from build123d import *

# Parameters (mm, degrees)
SM_BASE_FLANGE_1_DEPTH = 24
CUT_EXTRUDE_1_DEPTH    = 135.033577883
FILLET_1_R             = 10


# Sheet-metal steps are written as plain solids
with BuildPart() as part:
    # Sketch 1 → 基体-法兰1 (new, symmetric)
    with BuildSketch(Plane(origin=(0, 0, 0), x_dir=(0, 0, -1), z_dir=(1, 0, 0))):
        with BuildLine():
            Line((-125, 50), (-125, 16))
            ThreePointArc((-125, 16), (-120.313708499, 4.686291501), (-109, 0))
            Line((-109, 0), (109, 0))
            ThreePointArc((109, 0), (120.313708499, 4.686291501), (125, 16))
            Line((125, 16), (125, 50))
            Line((125, 50), (117, 50))
            Line((117, 50), (117, 16))
            ThreePointArc((117, 16), (114.656854249, 10.343145751), (109, 8))
            Line((109, 8), (-109, 8))
            ThreePointArc((-109, 8), (-114.656854249, 10.343145751), (-117, 16))
            Line((-117, 16), (-117, 50))
            Line((-117, 50), (-125, 50))
        make_face()
    extrude(amount=SM_BASE_FLANGE_1_DEPTH, both=True)

    # 草图6 → 切除-拉伸1 (cut, through all)
    with BuildSketch(Plane(origin=(0, 8, 0), x_dir=(1, 0, 0), z_dir=(0, 1, 0))):
        with BuildLine():
            Line((7.5, 77.5), (7.5, 72.5))
            ThreePointArc((7.5, 72.5), (0, 65), (-7.5, 72.5))
            Line((-7.5, 72.5), (-7.5, 77.5))
            ThreePointArc((-7.5, 77.5), (0, 85), (7.5, 77.5))
        make_face()
        with BuildLine():
            Line((7.5, 27.5), (7.5, 22.5))
            ThreePointArc((7.5, 22.5), (0, 15), (-7.5, 22.5))
            Line((-7.5, 22.5), (-7.5, 27.5))
            ThreePointArc((-7.5, 27.5), (0, 35), (7.5, 27.5))
        make_face()
        with BuildLine():
            Line((7.5, -22.5), (7.5, -27.5))
            ThreePointArc((7.5, -27.5), (0, -35), (-7.5, -27.5))
            Line((-7.5, -27.5), (-7.5, -22.5))
            ThreePointArc((-7.5, -22.5), (0, -15), (7.5, -22.5))
        make_face()
        with BuildLine():
            Line((7.5, -72.5), (7.5, -77.5))
            ThreePointArc((7.5, -77.5), (0, -85), (-7.5, -77.5))
            Line((-7.5, -77.5), (-7.5, -72.5))
            ThreePointArc((-7.5, -72.5), (0, -65), (7.5, -72.5))
        make_face()
    extrude(amount=-CUT_EXTRUDE_1_DEPTH, mode=Mode.SUBTRACT)

    # 圆角1
    fillet_1_edges = [part.edges().sort_by_distance(p)[0] for p in [
        (-24, 50, 121),
        (-24, 50, -121),
        (24, 50, 121),
        (24, 50, -121),
    ]]
    fillet(fillet_1_edges, radius=FILLET_1_R)


solid = part.part
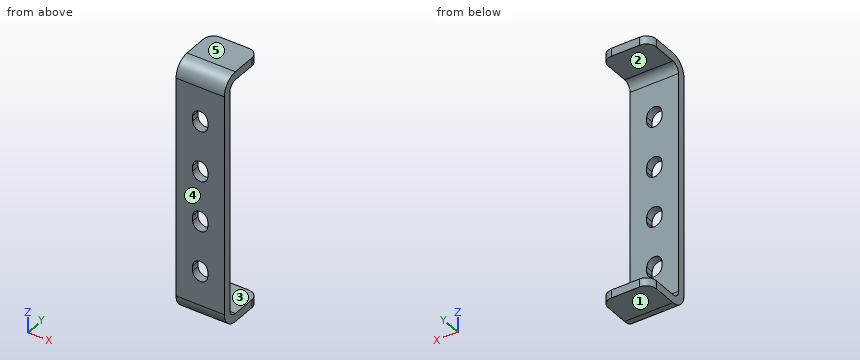
The listing builds one solid part. Answer for the finished solid, in the listing's coordinates (mm). Face numbers are marked on the shaded views. A direction names the side the tool comes from. Round coordinates to 2 decimals unless told otherwise and drop trailing zeros. Order: outer loops, then holes, each group sorted by start corner. A loop starts at its lowest first (then second) coordinate and runs counter-clockwise, first axis right, second up. Notation, with made-up numbers: (41, -4.5) -> (63, -4.5) arc R16 ccw to (63, 4.5) -> close; hole circle Ø1 at (-32.5, 66). An arc over 180 degrees is marked (long way). One line per item, written item: value.
Item 1: Straight lines are drawn through the part: L1, parallel to Z at x = -4, y = 18; L2, parallel to Z at x = 2.5, y = 2; L3, parallel to Y at x = 18, z = 97.5. For each, find the intervals that lie inside material, in ascending order.
Taken from the geometry:
L1: z = -125 to -117, 117 to 125
L2: z = -116.75 to -84.57, -65.43 to -34.57, -15.43 to 15.43, 34.57 to 65.43, 84.57 to 116.75
L3: y = 0 to 8
Item 2: Find section C-C, the plane z = -30. Give the vertices of the cut face in (x, y).
Taken from the geometry:
outline: (-24, 0) -> (-7.07, 0) -> (-7.07, 8) -> (-24, 8) -> close; (7.07, 0) -> (24, 0) -> (24, 8) -> (7.07, 8) -> close
Item 3: For a pull along Z with two mould halves and no side action, classify the marked faces 3, 4 and 5 as released by +Z, released by -Z, zero draft, split by the parting line, or undercut.
Taken from the geometry:
face 3: undercut
face 4: zero draft
face 5: released by +Z
Item 4: Given P1, Ø10, axis at x = -1, z = -24.5, coming from the +Y side; P2, Ø3, axis at x = 6.5, y = 9, coming from the +Z side (3 decimals); P3, Ø8, axis at x = -16, y = 10, coming from the +Z side; P4, Ø6, axis at x = -13.5, z = 21.5, coming from the +Y side, each flat-ended and moving along its own axis, determine where each tip first touches the part or whether it passes through.
Taken from the geometry:
P1: passes through
P2: stops at z = 124.025
P3: stops at z = 124.87
P4: stops at y = 8
Item 5: Find section A-A, the plane x = 0. Give the vertices of the cut face in (y, z).
Taken from the geometry:
outline: (0, -109) arc R16 ccw to (16, -125) -> (50, -125) -> (50, -117) -> (16, -117) arc R8 cw to (8, -109) -> (8, -85) -> (0, -85) -> close; (0, -65) -> (8, -65) -> (8, -35) -> (0, -35) -> close; (0, -15) -> (8, -15) -> (8, 15) -> (0, 15) -> close; (0, 35) -> (8, 35) -> (8, 65) -> (0, 65) -> close; (0, 85) -> (8, 85) -> (8, 109) arc R8 cw to (16, 117) -> (50, 117) -> (50, 125) -> (16, 125) arc R16 ccw to (0, 109) -> close
Item 6: For the marked faces 1 and 2, determine the directions among +Z, -Z, +X, -X, +Y, -Y from which every point of the face is accessible in a straight line to the end or side of a thin tool.
Taken from the geometry:
face 1: -Z, +X, -X, +Y, -Y
face 2: +X, -X, +Y
Item 7: Find section D-D, the plane z = -93.5. Give the vertices of the cut face in (x, y).
Taken from the geometry:
outline: (-24, 0) -> (24, 0) -> (24, 8) -> (-24, 8) -> close
Item 8: Find section B-B, the plane y = 23. Give the vertices of the cut face in (x, z).
Taken from the geometry:
outline: (-24, -125) -> (24, -125) -> (24, -117) -> (-24, -117) -> close; (-24, 117) -> (24, 117) -> (24, 125) -> (-24, 125) -> close
